from build123d import *

# Parameters (mm, degrees)
SKETCH1_W           = 31.75
SKETCH1_H           = 7.9375
BOSS_EXTRUDE1_DEPTH = 1.6
SKETCH2_R           = 1.5875
CUT_EXTRUDE1_DEPTH  = 17.441611891


with BuildPart() as part:
    # Sketch1 → Boss-Extrude1 (new body)
    with BuildSketch(Plane(origin=(0, 0, 0), x_dir=(1, 0, 0), z_dir=(0, 1, 0))):
        Rectangle(SKETCH1_W, SKETCH1_H)
    extrude(amount=BOSS_EXTRUDE1_DEPTH)

    # Sketch2 → Cut-Extrude1 (cut, through all)
    with BuildSketch(Plane(origin=(0, 1.6, 0), x_dir=(1, 0, 0), z_dir=(0, 1, 0))):
        with Locations(Location((-9.525, 0, 0), (0, 0, 270))):
            Circle(SKETCH2_R)
        with Locations(Location((9.525, 0, 0), (0, 0, 270))):
            Circle(SKETCH2_R)
        with BuildLine():
            Line((-15.875, 1.5875), (-15.875, -1.5875))
            ThreePointArc((-15.875, -1.5875), (-14.2875, 0), (-15.875, 1.5875))
        make_face()
        with BuildLine():
            Line((15.875, -1.5875), (15.875, 1.5875))
            ThreePointArc((15.875, 1.5875), (14.2875, 0), (15.875, -1.5875))
        make_face()
    extrude(amount=-CUT_EXTRUDE1_DEPTH, mode=Mode.SUBTRACT)


solid = part.part
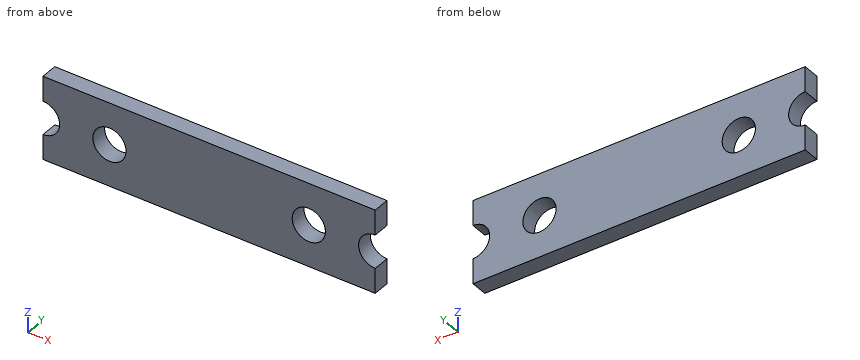
Geometry check sheet. Reference: the model listing, model coordinates, mm. Coordinates: 2 decimals unless noted, no trailing zeros. Order: outer loops, then holes, each group sorted by start corner. A loop starts at its lowest first (then second) coordinate and runs counter-clockwise, first axis right, second up. Notation, with made-up numbers: (51.5, 43.25) - (84.5, 43.25) arc R13 ccw to (84.5, 63.25) - close; hole circle Ø11 at (82.5, -7). An arc over 180 degrees is marked (long way). Answer in a Markdown table with one row per item. Add a question column.
1) Cross-section at A-A, the plane z = 0. Record the cut outline in (x, y).
2) Material ranges on line 1 along X through (y, z) = (0.85, 0); line 2 along X through (y, z) = (0.95, -0.75); line 3 along Z through (x, y) = (-10, 1.15), recorded low to high. Write a range as [from, to].
3) Cross-section at B-B, the plane y = 0.4. Record the cut outline in (x, z) (1 decimal), then the cut area to 3 significant figures.
Check result:
| question | item | result |
|---|---|---|
| 1 | outline | (-14.29, 0) - (-11.11, 0) - (-11.11, 1.6) - (-14.29, 1.6) - close; (-7.94, 0) - (7.94, 0) - (7.94, 1.6) - (-7.94, 1.6) - close; (11.11, 0) - (14.29, 0) - (14.29, 1.6) - (11.11, 1.6) - close |
| 2 | line 1 | x = [-14.29, -11.11], [-7.94, 7.94], [11.11, 14.29] |
| 2 | line 2 | x = [-14.48, -10.92], [-8.13, 8.13], [10.92, 14.48] |
| 2 | line 3 | z = [-3.97, -1.51], [1.51, 3.97] |
| 3 | outline | (-15.9, -4) - (15.9, -4) - (15.9, -1.6) arc R1.6 cw to (15.9, 1.6) - (15.9, 4) - (-15.9, 4) - (-15.9, 1.6) arc R1.6 cw to (-15.9, -1.6) - close; hole circle Ø3.2 at (-9.5, 0); hole circle Ø3.2 at (9.5, 0) |
| 3 | area | 228 mm² |
